For this review, take the finished solid that the model builds, in its own axes (mm). Give positions to 0.01 mm unless a question says otherwise; leave off trailing zeros. Order: outer loops, then holes, each group sorted by start corner. A loop starts at its lowest first (then second) coordinate and runs counter-clockwise, first axis right, second up.
from build123d import *


with BuildPart() as f1:
    # F0 (on Right) → F1 (revolve)
    with BuildSketch(Plane.YZ):
        Polygon((2, 6), (0, 6), (-6, 6), (-6, 5), (-7, 5), (-7, 6), (-12, 6), (-12, 0), (0, 0), (65.5, 0), (65.5, 6), (63, 6), (63, 5), (62, 5), (62, 6), (57, 6), (57, 5), (56, 5), (56, 6), (30, 6), (29, 6), (11, 6), (11, 5), (10, 5), (10, 6), (3, 6), (3, 5), (2, 5), align=None)
    revolve(axis=Axis((0, 32.75, 0), (0, 1, 0)))


solid = f1.part
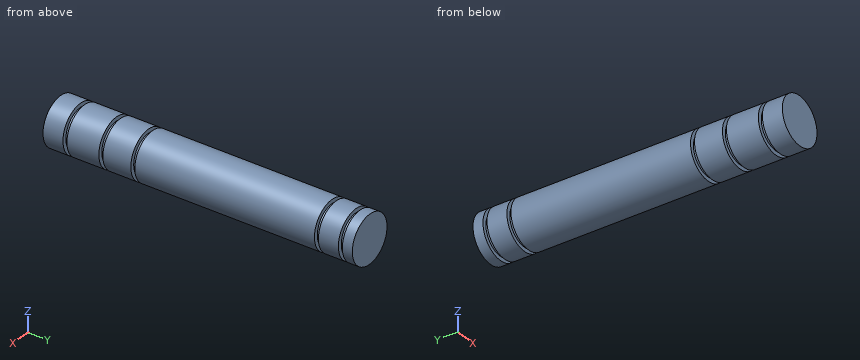
1) We need section A-A on y = -2.5. Give the boundary of the cut face in (x, z), then the cut area to 3 significant figures.
Answer sheet:
outline: circle Ø12 at (0, 0)
area: 113 mm2
2) To check wall thickness, follow line 1 (Y direction, x = 4.75, z = -3.25); line 2 (X direction, y = 17, z = 2.5); line 3 (X direction, y = 16, z = 1.75). State the ranges of each line that lie inside material, in increasing order.
Answer sheet:
line 1: y = -12 to -7, -6 to 2, 3 to 10, 11 to 56, 57 to 62, 63 to 65.5
line 2: x = -5.45 to 5.45
line 3: x = -5.74 to 5.74
3) Clearance check with flat-ended pins moving along their axes: pin 1 (6 mm diameter, centred on y = 37.5, z = 3.5, fed in from +X); pin 2 (5 mm diameter, centred on y = 2.5, z = -3, fed in from -X). State where each tip first meets the part, or that it passes through.
Answer sheet:
pin 1: stops at x = 5.98
pin 2: stops at x = -5.97
